```python
from build123d import *

# Parameters (mm, degrees)
BOSS_EXTRUDE1_DEPTH      = 52
SKETCH2_R                = 2.5
SKETCH2_R_2              = 1.5
CUT_EXTRUDE1_DEPTH       = 26
BOSS_EXTRUDE2_DEPTH      = 11.5
BOSS_EXTRUDE2_DEPTH_BACK = 11.5


with BuildPart() as part:
    # Sketch1 → Boss-Extrude1 (new body)
    with BuildSketch(Plane(origin=(0, 0, 0), x_dir=(1, 0, 0), z_dir=(0, 1, 0))):
        with BuildLine():
            Line((13.5, 0), (13.5, 12.2))
            ThreePointArc((13.5, 12.2), (12.914213562, 13.614213562), (11.5, 14.2))
            Line((11.5, 14.2), (-11.5, 14.2))
            ThreePointArc((-11.5, 14.2), (-12.914213562, 13.614213562), (-13.5, 12.2))
            Line((-13.5, 12.2), (-13.5, 0))
            Line((-13.5, 0), (-12, 0))
            Line((-12, 0), (-12, 12.2))
            ThreePointArc((-12, 12.2), (-11.853553391, 12.553553391), (-11.5, 12.7))
            Line((-11.5, 12.7), (11.5, 12.7))
            ThreePointArc((11.5, 12.7), (11.853553391, 12.553553391), (12, 12.2))
            Line((12, 12.2), (12, 0))
            Line((12, 0), (13.5, 0))
        make_face()
    extrude(amount=BOSS_EXTRUDE1_DEPTH)

    # Sketch2 → Cut-Extrude1 (cut, symmetric)
    with BuildSketch(Plane(origin=(0, 0, 0), x_dir=(0, 0, -1), z_dir=(1, 0, 0))):
        with Locations((5, 5)):
            Circle(SKETCH2_R)
        with Locations((5.917597774, 46.082402226)):
            Circle(SKETCH2_R_2)
        with Locations((4.5, 35.5)):
            Circle(SKETCH2_R_2)
        with BuildLine():
            Line((12.2, 45.5), (11.633558293, 47.613989232))
            ThreePointArc((11.633558293, 47.613989232), (4.857073421, 51.904193317), (0.028729372, 45.5))
            Line((0.028729372, 45.5), (-2.330829718, 45.5))
            Line((-2.330829718, 45.5), (-2.330829718, 58.046352069))
            Line((-2.330829718, 58.046352069), (16.335993039, 58.046352069))
            Line((16.335993039, 58.046352069), (16.335993039, 45.5))
            Line((16.335993039, 45.5), (12.2, 45.5))
        make_face()
        with BuildLine():
            Line((0, 5), (0, 0))
            Line((0, 0), (5, 0))
            ThreePointArc((5, 0), (1.464466094, 1.464466094), (0, 5))
        make_face()
    extrude(amount=CUT_EXTRUDE1_DEPTH, both=True, mode=Mode.SUBTRACT)

    # Sketch4 → Boss-Extrude2 (add, two sides)
    with BuildSketch(Plane(origin=(0, 0, 0), x_dir=(0, 0, -1), z_dir=(1, 0, 0))) as boss_extrude2_sk:
        with BuildLine():
            Line((12.694645471, 0), (14.2, 0))
            ThreePointArc((14.2, 0), (15.225683929, -6.216635866), (17.200004735, -12.2))
            Line((17.200004735, -12.2), (15.579003919, -12.2))
            ThreePointArc((15.579003919, -12.2), (13.680583201, -6.207865902), (12.694645471, 0))
        make_face()
    extrude(amount=BOSS_EXTRUDE2_DEPTH)
    extrude(boss_extrude2_sk.sketch, amount=-BOSS_EXTRUDE2_DEPTH_BACK)


solid = part.part
```
For this review, take the finished solid that the model builds, in its own axes (mm). A direction names the side the tool comes from. Give positions to 0.01 mm unless a question says otherwise; leave off trailing zeros. Write each loop counter-clockwise with the first axis right and the second up, starting at its lowest first coordinate (ties: lowest second). Pieces come first, ordered by that corner, then holes. Notation, with made-up numbers: M -14.5,-5.75 L 12.5,-5.75 A19 ccw 12.5,22.25 Z; hole C -0.75,-8.75 d3. An arc over 180 degrees is marked long. One line per item, written item: value.
1) Take a section at D-D, the plane z = -13.5. Write out the cut boundary in (x, y), then the cut area to 3 significant figures.
Results are:
outline: M -13.02,0 L -11.5,0 L -11.5,-5.41 L 11.5,-5.41 L 11.5,0 L 13.02,0 L 13.02,45.5 L -13.02,45.5 Z
area: 1,310 mm²
2) For line 1 (X direction, y = 33, z = -11); line 2 (Z direction, x = -6, y = 10); line 3 (Z direction, x = 13.15, y = 5), list the stretches that pass through material, from the lowest coordinate up. Write a range as from..to.
Results are:
line 1: x = -13.5..-12, 12..13.5
line 2: z = -14.2..-12.7
line 3: z = -13.33..-7.5, -2.5..0
3) Take a section at A-A, the plane y = 35.5. Write out the cut boundary in (x, z), then the cut area to 3 significant figures.
Results are:
outline: M -13.5,-12.2 A2 ccw -11.5,-14.2 L 11.5,-14.2 A2 ccw 13.5,-12.2 L 13.5,-6 L 12,-6 L 12,-12.2 A0.5 cw 11.5,-12.7 L -11.5,-12.7 A0.5 cw -12,-12.2 L -12,-6 L -13.5,-6 Z; M -13.5,-3 L -12,-3 L -12,0 L -13.5,0 Z; M 12,-3 L 13.5,-3 L 13.5,0 L 12,0 Z
area: 68.0 mm²
4) The part is to be moulded in two halves that separate along Z. For faces 1 (the flat face through (-13, 25, 0)), 2 (the cylindrical face through (12.74, 47.57, -5.72)), 3 (the cylindrical face through (-12.76, 51.925, -4.979)), say which applies: +Z half, -Z half, draft (parallel to the pull), parting line (faces both ways), or undercut.
Results are:
face 1: +Z half
face 2: undercut
face 3: parting line
5) For faces 4 (the cylindrical face through (-12.9, 22.43, -13.63)), 5 (the cylindrical face through (12.74, 34.17, -5.19)), 6 (the flat face through (-11.5, -6, -15)), 7 (the flat face through (0, 22, -12.7)), 8 (the flat face through (0, 45.5, -13)), list the 3-axis set-ups (+Z, -Z, +X, -X, +Y, -Y) from which the entire face can be reached by the end or side of a thin tool; tool diameter is ignored.
Results are:
face 4: -Z, -X, +Y, -Y
face 5: +X, -X
face 6: +Z, -Z, -X, -Y
face 7: +Z, +Y, -Y
face 8: -Z, +X, -X, +Y
6) For P1, Ø2, axis at x = -2, z = -13, coming from the +Y side; P2, Ø3.5, axis at y = -6.5, z = -14, coming from the +X side; P3, Ø0.6, axis at x = -13, z = -8, coming from the -Y side, all flat-tipped, find the tip position at first contact; note any pin that passes through.
Results are:
P1: stops at y = 45.5
P2: stops at x = 11.5
P3: stops at y = 0
7) Take a section at C-C, the plane z = -9.5. Write out the cut boundary in (x, y), then the cut area to 3 significant figures.
Results are:
outline: M -13.5,0 L -12,0 L -12,50.79 L -13.5,50.79 Z; M 12,0 L 13.5,0 L 13.5,50.79 L 12,50.79 Z
area: 152 mm²
